```python
from build123d import *

# Parameters (mm, degrees)
F2_DEPTH = 4
F1_R     = 1
F3_DEPTH = 22.2
F5_R     = 0.49999


# Not quite as in the source:
# - a fillet or chamfer is up to 0.001 mm smaller than in the source, because OpenCascade refuses the exact size


with BuildPart() as f2:
    # F0 (on Top) → F2 (new body)
    with BuildSketch(Plane.XY):
        Polygon((0, 2), (0, 0), (7.9, 0), (7.9, 18.2000004202), (12.1, 18.2000004202), (12.1, 0), (20, 0), (20, 2), (14, 2), (14, 20.2), (6, 20.2), (6, 2), align=None)
    extrude(amount=F2_DEPTH)


with BuildPart() as f3:
    # F1 (on Front) → F3 (new body)
    with BuildSketch(Plane.XZ):
        with Locations((4, 2)):
            Circle(F1_R)
    extrude(amount=-F3_DEPTH)


with BuildPart() as f3b:
    # F1 (on Front) → F3, piece 2 (new body)
    with BuildSketch(Plane.XZ):
        with Locations((16, 2)):
            Circle(F1_R)
    extrude(amount=-F3_DEPTH)


with BuildPart() as f2_1:
    add(f2.part)

    # F4: cut F3, F3b
    add(f3.part, mode=Mode.SUBTRACT)
    add(f3b.part, mode=Mode.SUBTRACT)

    # F5 (radius 0.5 in the source; OpenCascade refuses exactly that, so slightly less here)
    f5_edges = [f2_1.edges().sort_by_distance(p)[0] for p in [
        (7.9, 0, 2),
        (12.1, 0, 2),
        (14, 20.2, 2),
        (7.9, 18.2, 2),
        (12.1, 18.2, 2),
        (6, 20.2, 2),
        (6, 2, 2),
        (14, 2, 2),
        (3, 2, 2),
        (15, 2, 2),
        (3, 0, 2),
        (15, 0, 2),
    ]]
    fillet(f5_edges, radius=F5_R)


solid = f2_1.part
```
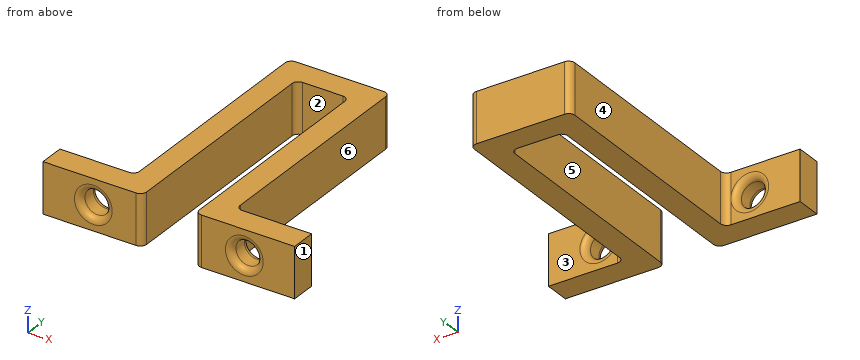
CAD build for the part. Positions are in the model's coordinates, mm. Face numbers are marked on the shaded views. A direction names the side the tool comes from. Coordinates: 2 decimals unless noted, no trailing zeros. Write each loop counter-clockwise with the first axis right and the second up, starting at its lowest first coordinate (ties: lowest second). Pieces come first, ordered by that corner, then holes. Notation, with made-up numbers: (7, 13) -> (24, 13) arc R7 cw to (24, 19) -> close; hole circle Ø7 at (2, 87.5). An arc over 180 degrees is marked (long way). Return JSON: item names as keys, results as strings. Group by question number.
Q1. Drill centre lines: line 1 (X direction, y = 17.75, z = 1.6); line 2 (Z direction, x = 16, y = 1); line 3 (Y direction, x = 18.5, z = 0.5). Where is each one in solid material? Low to high.
Q2. Flat gauge pins, fed straight in: pin 1 (10 mm diameter, centred on x = 5.5, y = 7, fed in from -Z); pin 2 (2 mm diameter, centred on x = 3.5, z = 2.5, fed in from +Y); pin 3 (1.5 mm diameter, centred on x = 14.5, z = 3, fed in from +Y); pin 4 (1.2 mm diameter, centred on y = 9.5, z = 3, fed in from +X). Where does each tip first touch, or does it go through?
Q3. Which spindle directions (+Z, -Z, +X, -X, +Y, -Y) get a long thin tool onto all of the face, cutting with end or side? Do the marked faces 4, 5 and 6. Say none if no direction does.
Q4. Cut at C-C, the plane z = 2. State how many separate pieces and enclosed holes the cut face has, then the cut area to 3 significant figures.
Q5. Pull direction X, two halves, no side cores. Call the marked faces 1, 2 and 3: released by +X, released by -X, zero draft, split by the parting line, or undercut.
Q6. Cut at A-A, the plane y = 7.25. Give the cut face in (x, z), then the cut area to 3 significant figures.
Q7. Cut at B-B, the plane x = 4. Give the cut face in (y, z).
Q8. Cut at D-D, the plane x = 11. Give the cut face in (y, z), then the cut area to 3 significant figures.
Returned:
{
 "1": {"line 1": "x = 6 to 7.9, 12.1 to 14", "line 2": "z = 0 to 1, 3 to 4", "line 3": "y = 0 to 2"},
 "2": {"pin 1": "stops at z = 0", "pin 2": "stops at y = 2", "pin 3": "stops at y = 20.13", "pin 4": "stops at x = 14"},
 "3": {"face 4": "+Z, -Z, -X, +Y", "face 5": "+Z, -Z, -Y", "face 6": "+Z, -Z, +X, +Y"},
 "4": {"separate pieces": "3", "enclosed holes": "0", "area": "101 mm2"},
 "5": {"face 1": "released by +X", "face 2": "undercut", "face 3": "zero draft"},
 "6": {"outline": "(6, 0) -> (7.9, 0) -> (7.9, 4) -> (6, 4) -> close; (12.1, 0) -> (14, 0) -> (14, 4) -> (12.1, 4) -> close", "area": "15.2 mm2"},
 "7": {"outline": "(0, 0) -> (2, 0) -> (2, 0.5) arc R0.5 ccw to (1.5, 1) -> (0.5, 1) arc R0.5 ccw to (0, 0.5) -> close; (0, 3.5) arc R0.5 ccw to (0.5, 3) -> (1.5, 3) arc R0.5 ccw to (2, 3.5) -> (2, 4) -> (0, 4) -> close"},
 "8": {"outline": "(18.2, 0) -> (20.2, 0) -> (20.2, 4) -> (18.2, 4) -> close", "area": "8.00 mm2"}
}
